```python
from build123d import *

# Parameters (mm, degrees)
F0_W     = 14
F0_H     = 14
F1_DEPTH = 3
F2_W     = 14
F2_H     = 14
F3_DEPTH = 4
F4_ANGLE = -90
F5_ANGLE = -90


# Not quite as in the source:
# - a feature names something its author has since deleted; it is built from what else it names


with BuildPart() as f1:
    # F0 (on Top) → F1 (new body)
    with BuildSketch(Plane.XY):
        Rectangle(F0_W, F0_H)
        with BuildLine():
            ThreePointArc((1.9485571585, 1.125), (2.1733331092, 0.5823428515), (2.25, 0))
            ThreePointArc((2.25, 0), (2.1733331092, -0.5823428515), (1.9485571585, -1.125))
            ThreePointArc((1.9485571585, -1.125), (-2.25, 0), (1.9485571585, 1.125))
        make_face(mode=Mode.SUBTRACT)
    extrude(amount=F1_DEPTH)

    # F2 (on face) → F3 (join)
    with BuildSketch(Plane.XY.offset(3)):
        Rectangle(F2_W, F2_H)
        with BuildLine():
            ThreePointArc((4.3734282891, 2.525), (4.8779254228, 1.3070361778), (5.05, 0))
            ThreePointArc((5.05, 0), (4.8779254228, -1.3070361778), (4.3734282891, -2.525))
            ThreePointArc((4.3734282891, -2.525), (2.525, -4.3734282891), (0, -5.05))
            ThreePointArc((0, -5.05), (-2.525, -4.3734282891), (-4.3734282891, -2.525))
            ThreePointArc((-4.3734282891, -2.525), (-5.05, 0), (-4.3734282891, 2.525))
            ThreePointArc((-4.3734282891, 2.525), (-2.525, 4.3734282891), (0, 5.05))
            ThreePointArc((0, 5.05), (2.525, 4.3734282891), (4.3734282891, 2.525))
        make_face(mode=Mode.SUBTRACT)
        with BuildLine():
            Line((-4.3734282891, -2.525), (-4.3734282891, 2.525))
            ThreePointArc((-4.3734282891, 2.525), (-5.05, 0), (-4.3734282891, -2.525))
        make_face()
        with BuildLine():
            Line((-4.3734282891, 2.525), (0, 5.05))
            ThreePointArc((0, 5.05), (-2.525, 4.3734282891), (-4.3734282891, 2.525))
        make_face()
        with BuildLine():
            Line((0, 5.05), (4.3734282891, 2.525))
            ThreePointArc((4.3734282891, 2.525), (2.525, 4.3734282891), (0, 5.05))
        make_face()
        with BuildLine():
            ThreePointArc((4.3734282891, -2.525), (4.8779254228, -1.3070361778), (5.05, 0))
            ThreePointArc((5.05, 0), (4.8779254228, 1.3070361778), (4.3734282891, 2.525))
            Line((4.3734282891, 2.525), (4.3734282891, -2.525))
        make_face()
        with BuildLine():
            ThreePointArc((0, -5.05), (2.525, -4.3734282891), (4.3734282891, -2.525))
            Line((4.3734282891, -2.525), (0, -5.05))
        make_face()
        with BuildLine():
            ThreePointArc((-4.3734282891, -2.525), (-2.525, -4.3734282891), (0, -5.05))
            Line((0, -5.05), (-4.3734282891, -2.525))
        make_face()
    extrude(amount=F3_DEPTH)


with BuildPart() as f1_1:
    # F4: moved
    add(f1.part.rotate(Axis((0, -7, 0), (-1, 0, 0)), F4_ANGLE))


with BuildPart() as f1_2:
    # F5: moved
    add(f1_1.part.rotate(Axis((7, -7, 7), (0, 0, -1)), F5_ANGLE))


solid = f1_2.part
```
Read the model definition and answer for the solid it produces. Units are mm, in the model's axes. A direction names the side the tool comes from. Give positions to 0.01 mm unless a question says otherwise; leave off trailing zeros. Write each loop counter-clockwise with the first axis right and the second up, starting at its lowest first coordinate (ties: lowest second). Pieces come first, ordered by that corner, then holes. Notation, with made-up numbers: (27, 15) -> (43, 15) arc R17 ccw to (43, 39) -> close; hole circle Ø11 at (22, 16.25). An arc over 180 degrees is marked (long way). Answer in a Markdown table with one row per item.
1) Straight lines are drawn through the part: line 1 (Y direction, x = 8.9, z = 7); line 2 (Y direction, x = 13.75, z = 9.25); line 3 (Z direction, x = 8.35, y = -14). For each, find the intervals that lie inside material, in ascending order. Write a range as [from, to].
Results list:
| item | result |
|---|---|
| line 1 | [-21, -16.25], [-11.75, -7] |
| line 2 | [-21, -18.37], [-9.63, -7] |
| line 3 | [0, 4.75], [9.25, 14] |
2) Determine the mould class of faces 3 (the flat face through (14, -19, 7)), 4 (the flat face through (10, -14, 0)), 5 (the flat face through (11.97, -16.22, 10.77)), 6 (the flat face through (10, -14, 14)) for opening direction Z: released by +Z, released by -Z, zero draft, split by the parting line, or undercut.
Results list:
| item | result |
|---|---|
| face 3 | zero draft |
| face 4 | released by -Z |
| face 5 | undercut |
| face 6 | released by +Z |
3) Section C-C on y = -14.5 is taken. Give the vertices of the cut face in (x, z), plus the area to 3 significant figures.
Results list:
| item | result |
|---|---|
| outline | (7, 0) -> (14, 0) -> (14, 2.24) -> (10, 2.24) -> (10, 4.81) -> (7, 4.81) -> close; (7, 9.19) -> (10, 9.19) -> (10, 11.76) -> (14, 11.76) -> (14, 14) -> (7, 14) -> close |
| area | 46.7 mm^2 |
4) A tool of negligible diameter and unlimited length cuts with its end or side. For faces 1 (the flat face through (7, -16, 9)), 2 (the flat face through (12, -18.373, 7)), from which of +Z, -Z, +X, -X, +Y, -Y can it reach the whole face along a straight path? Write none if from no direction.
Results list:
| item | result |
|---|---|
| face 1 | +Z, -Z, -X, +Y, -Y |
| face 2 | +X |
5) Section A-A on z = 5.5 is taken. Give the vertices of the cut face in (x, y).
Results list:
| item | result |
|---|---|
| outline | (7, -21) -> (14, -21) -> (14, -18.37) -> (10, -18.37) -> (10, -15.68) -> (7, -15.68) -> close; (7, -12.32) -> (10, -12.32) -> (10, -9.63) -> (14, -9.63) -> (14, -7) -> (7, -7) -> close |
6) Section B-B on x = 8.75 is taken. Give the vertices of the cut face in (y, z) (3 decimals).
Results list:
| item | result |
|---|---|
| outline | (-21, 0) -> (-7, 0) -> (-7, 14) -> (-21, 14) -> close; hole circle Ø4.5 at (-14, 7) |
7) Each of these flat-tipped pins is pushed along its axis until it touches: pin 1 Ø1 at (x, y) = (12.5, -12) entering from -Z; pin 2 Ø4 at (y, z) = (-14, 7) entering from -X. Where does it stop, or does it pass through?
Results list:
| item | result |
|---|---|
| pin 1 | z = 0 |
| pin 2 | through |
8) Section D-D on x = 11 is taken. Give the vertices of the cut face in (y, z) (3 decimals).
Results list:
| item | result |
|---|---|
| outline | (-21, 0) -> (-7, 0) -> (-7, 14) -> (-21, 14) -> close; hole (-18.373, 4.475) -> (-14, 1.95) -> (-9.627, 4.475) -> (-9.627, 9.525) -> (-14, 12.05) -> (-18.373, 9.525) -> close |
